```python
from build123d import *

# Parameters (mm, degrees)
BOSS_EXTRUDE5_DEPTH          = 2.760049195
CHAMFER1_SIZE                = 1.510362865
CHAMFER1_SIZE2               = 0.926037145
BOSS_EXTRUDE6_DEPTH          = 24
BOSS_EXTRUDE7_DEPTH          = 5
BOSS_EXTRUDE8_DEPTH          = 6
BOSS_EXTRUDE9_DEPTH          = 4
SKETCH28_W                   = 2.760049196
SKETCH28_H                   = 4
CUT_EXTRUDE3_DEPTH           = 8.878692186
BOSS_EXTRUDE10_DEPTH         = 4
SKETCH45_W                   = 2.760049196
SKETCH45_H                   = 4
CUT_EXTRUDE4_DEPTH           = 0.7448337
BOSS_EXTRUDE11_DEPTH         = 5
F_4_0_4_DIAMETER_HOLE2_D     = 4
F_4_0_4_DIAMETER_HOLE2_DEPTH = 2.760049195
SKETCH58_W                   = 2.6375
SKETCH58_H                   = 10
SKETCH60_W                   = 2.6375
SKETCH60_H                   = 38
HOLE6_D                      = 5.275
HOLE6_DEPTH                  = 46
F_3_0_3_DIAMETER_HOLE2_D     = 3
F_3_0_3_DIAMETER_HOLE2_DEPTH = 35
FILLET3_R                    = 2
FILLET4_R                    = 3


with BuildPart() as part:
    # Sketch17 → Boss-Extrude5 (new body)
    with BuildSketch(Plane(origin=(57.196631886, 0, 0), x_dir=(0, -1, 0), z_dir=(-1, 0, 0))):
        with BuildLine():
            Line((-38, -27.633835998), (-14, -27.633835998))
            ThreePointArc((-14, -27.633835998), (-12, -25.633835998), (-10, -27.633835998))
            Line((-10, -27.633835998), (-10, -9.028355512))
            Line((-10, -9.028355512), (-42, -9.028355512))
            Line((-42, -9.028355512), (-42, -27.633835998))
            ThreePointArc((-42, -27.633835998), (-40, -25.633835998), (-38, -27.633835998))
        make_face()
    extrude(amount=-BOSS_EXTRUDE5_DEPTH)

    # Chamfer1
    chamfer1_edges = [part.edges().sort_by_distance(p)[0] for p in [
        (59.956681082, 26, -9.028355512),
    ]]
    chamfer1_side = [part.faces().sort_by_distance(p)[0] for p in [
        (59.956681082, 26, -18.148814744),
    ]]
    chamfer(chamfer1_edges, length=CHAMFER1_SIZE, length2=CHAMFER1_SIZE2, reference=chamfer1_side[0])

    # Sketch18 → Boss-Extrude6 (add)
    with BuildSketch(Plane(origin=(0, 38, 0), x_dir=(1, 0, 0), z_dir=(0, 1, 0))):
        with BuildLine():
            Line((57.196631886, 27.633835998), (59.956681082, 27.633835998))
            Line((59.956681082, 27.633835998), (59.956681082, 37.518663649))
            ThreePointArc((59.956681082, 37.518663649), (52.044420209, 35.109942461), (57.196631886, 28.639971463))
            Line((57.196631886, 28.639971463), (57.196631886, 27.633835998))
        make_face()
    extrude(amount=-BOSS_EXTRUDE6_DEPTH)

    # Sketch19 → Boss-Extrude7 (add)
    with BuildSketch(Plane(origin=(0, 35, 0), x_dir=(1, 0, 0), z_dir=(0, 1, 0))):
        with BuildLine():
            Line((57.196631886, 15.88036097), (57.196631886, 23.207838196))
            add(Edge.make_bspline(
                [(55.511713205, 21.752088745), (56.732163203, 22.065636669), (57.196631886, 23.207838196)],
                knots=[0, 0, 0, 1, 1, 1], degree=2))
            ThreePointArc((55.511713205, 21.752088745), (53.511713205, 19.752088745), (55.511713205, 17.752088745))
            add(Edge.make_bspline(
                [(57.196631886, 15.88036097), (56.909946197, 17.31678815), (55.511713205, 17.752088745)],
                knots=[0, 0, 0, 1, 1, 1], degree=2))
        make_face()
    extrude(amount=-BOSS_EXTRUDE7_DEPTH)

    # Sketch20 → Boss-Extrude8 (add)
    with BuildSketch(Plane.XZ.offset(-10)):
        with BuildLine():
            Line((57.196631886, -28.639971463), (57.196631886, -9.028355512))
            Line((57.196631886, -9.028355512), (59.030643937, -9.028355512))
            Line((59.030643937, -9.028355512), (59.956681082, -10.538718377))
            Line((59.956681082, -10.538718377), (59.956681082, -37.518663649))
            ThreePointArc((59.956681082, -37.518663649), (52.044420209, -35.109942461), (57.196631886, -28.639971463))
        make_face()
    extrude(amount=BOSS_EXTRUDE8_DEPTH)

    # Sketch21 → Boss-Extrude9 (add)
    with BuildSketch(Plane.XZ.offset(-4)):
        Polygon((57.196631886, -27.895137764), (57.196631886, -9.028355512), (59.030643937, -9.028355512), (59.956681082, -10.538718377), (59.956681082, -27.895137764), (59.956681082, -28.639971463), (59.956681082, -37.518663649), (57.196631886, -37.518663649), (57.196631886, -28.639971463), align=None)
    extrude(amount=BOSS_EXTRUDE9_DEPTH)

    # Sketch28 → Cut-Extrude3 (cut)
    with BuildSketch(Plane(origin=(0, 0, -37.518663649), x_dir=(-1, 0, 0), z_dir=(0, 0, -1))):
        with Locations((-58.576656484, 2)):
            Rectangle(SKETCH28_W, SKETCH28_H)
    extrude(amount=-CUT_EXTRUDE3_DEPTH, mode=Mode.SUBTRACT)

    # Sketch36 → Boss-Extrude10 (add)
    with BuildSketch(Plane(origin=(0, 42, 0), x_dir=(1, 0, 0), z_dir=(0, 1, 0))):
        with BuildLine():
            Line((59.956681082, 37.518663649), (59.956681082, 10.538718377))
            Line((59.956681082, 10.538718377), (59.030643937, 9.028355512))
            Line((59.030643937, 9.028355512), (57.196631886, 9.028355512))
            Line((57.196631886, 9.028355512), (57.196631886, 28.639971463))
            ThreePointArc((57.196631886, 28.639971463), (52.044420209, 35.109942461), (59.956681082, 37.518663649))
        make_face()
    extrude(amount=BOSS_EXTRUDE10_DEPTH)

    # Sketch45 → Cut-Extrude4 (cut)
    with BuildSketch(Plane(origin=(0, 0, -28.639971463), x_dir=(-1, 0, 0), z_dir=(0, 0, -1))):
        with Locations((-58.576656484, 2)):
            Rectangle(SKETCH45_W, SKETCH45_H)
    extrude(amount=-CUT_EXTRUDE4_DEPTH, mode=Mode.SUBTRACT)

    # Sketch55 → Boss-Extrude11 (add)
    with BuildSketch(Plane(origin=(0, 46, 0), x_dir=(1, 0, 0), z_dir=(0, 1, 0))):
        Polygon((59.956681082, 10.538718377), (59.030643937, 9.028355512), (57.196631886, 9.028355512), (57.196631886, 27.895137764), (59.956681082, 27.895137764), align=None)
    extrude(amount=BOSS_EXTRUDE11_DEPTH)

    # Ø4.0 (4) Diameter Hole2
    with Locations(Plane.ZY.offset(-57.196631886)):
        with Locations((-22.895137764, 6), (-14.028355512, 6), (-14.028355512, 46), (-22.895137764, 46)):
            Hole(F_4_0_4_DIAMETER_HOLE2_D / 2, depth=F_4_0_4_DIAMETER_HOLE2_DEPTH)

    # Sketch58 → Hole4 (revolve, cut)
    with BuildSketch(Plane(origin=(56.81904117, 10, -33.625693603), x_dir=(0, 0, 1), z_dir=(1, 0, 0))):
        with Locations((1.31875, 5)):
            Rectangle(SKETCH58_W, SKETCH58_H)
    revolve(axis=Axis((56.81904117, -100, -33.625693603), (0, 1, 0)), mode=Mode.SUBTRACT)

    # Sketch60 → Hole5 (revolve, cut)
    with BuildSketch(Plane(origin=(56.81904117, 38, -33.625693603), x_dir=(0, 0, 1), z_dir=(1, 0, 0))):
        with Locations((1.31875, 19)):
            Rectangle(SKETCH60_W, SKETCH60_H)
    revolve(axis=Axis((56.81904117, -72, -33.625693603), (0, 1, 0)), mode=Mode.SUBTRACT)

    # Hole6
    with Locations(Plane(origin=(0, 46, 0), x_dir=(1, 0, 0), z_dir=(0, 1, 0))):
        with Locations((56.81904117, 33.625693603)):
            Hole(HOLE6_D / 2, depth=HOLE6_DEPTH)

    # Ø3.0 (3) Diameter Hole2
    with Locations(Plane(origin=(0, 35, 0), x_dir=(1, 0, 0), z_dir=(0, 1, 0))):
        with Locations((55.511713205, 19.752088745)):
            Hole(F_3_0_3_DIAMETER_HOLE2_D / 2, depth=F_3_0_3_DIAMETER_HOLE2_DEPTH)

    # Fillet3
    fillet3_edges = [part.edges().sort_by_distance(p)[0] for p in [
        (58.576656484, 46, -27.895137764),
        (58.576656484, 4, -27.895137764),
        (57.196631886, 26, -28.639971463),
    ]]
    fillet(fillet3_edges, radius=FILLET3_R)

    # Fillet4
    fillet4_edges = [part.edges().sort_by_distance(p)[0] for p in [
        (59.956681082, 26, -37.518663649),
        (59.956681082, 7, -37.518663649),
        (59.956681082, 44, -37.518663649),
    ]]
    fillet(fillet4_edges, radius=FILLET4_R)


solid = part.part
```
Work out the finished part from the listing and answer in its coordinate system (mm). A direction names the side the tool comes from. Round coordinates to 2 decimals unless told otherwise and drop trailing zeros. Write each loop counter-clockwise with the first axis right and the second up, starting at its lowest first coordinate (ties: lowest second). Pieces come first, ordered by that corner, then holes. Notation, with made-up numbers: (54, -10.5) -> (76, -10.5) arc R23 cw to (76, 1.5) -> close; hole circle Ø2 at (46.25, 30.25). An arc over 180 degrees is marked (long way). Write each question's results on one line, items separated by ' | '.
Q1. Straight lines are drawn through the part: line 1 along Y through (x, z) = (58.75, -31.5); line 2 along X through (y, z) = (20, -21.5); line 3 along Y through (x, z) = (59.25, -26). For each, find the intervals that lie inside material, in ascending order. Write a range as [from, to].
Data:
line 1: [4, 10], [14, 38], [42, 46] | line 2: [57.2, 59.96] | line 3: [0, 10.85], [13.15, 38.85], [41.15, 51]
Q2. Which of the six approach directions +Z, -Z, +X, -X, +Y, -Y give full straight-line access (tool end or side, diameter ignored) to faces 5 (the flat face through (59, 0, -18)), 6 (the flat face through (59, 1, -27.895)), 7 (the flat face through (54, 14, -33)), 8 (the flat face through (59, 49, -27.895))?
Data:
face 5: +Z, -Z, +X, -X, -Y | face 6: -Z, +X, -X, -Y | face 7: -Z, +X, -X | face 8: -Z, +X, -X, +Y
Q3. Section D-D, the plane x = 54.75 is taken. Give the number of separate pieces and of enclosed holes in the cut face, then the cut area to 3 significant figures.
Data:
separate pieces: 8 | enclosed holes: 0 | area: 204 mm^2
Q4. Flat-ended cylindrical pins translate along their axes: P1, Ø3, axis at x = 55, z = -20, coming from the +Y side; P2, Ø3.5, axis at y = 46, z = -22.9, coming from the +X side (1 decimal); P3, Ø6, axis at y = 34, z = -23.5, coming from the -X side; P4, Ø1.5, axis at y = 37.5, z = -15.5, coming from the -X side. Find the tip coordinate at first contact, or state that the pin passes through.
Data:
P1: y = 35 | P2: through | P3: x = 53.66 | P4: x = 57.2
Q5. Section A-A, the plane y = 6 is taken. Write down the section's boundary in (x, z) (1 decimal).
Data:
outline: (57.2, -38.6) arc R3 ccw to (60, -35.6) -> (60, -24.9) -> (57.2, -24.9) -> (57.2, -28.6) arc R5 ccw (long way) to start; (57.2, -20.9) -> (60, -20.9) -> (60, -16) -> (57.2, -16) -> close; (57.2, -12) -> (60, -12) -> (60, -10.5) -> (59, -9) -> (57.2, -9) -> close; hole circle Ø5.3 at (56.8, -33.6)
Q6. Determine the mould class of faces 1 (the cylindrical face through (55.214, 6.958, -35.719)), 2 (the flat face through (54, 42, -33)), 3 (the flat face through (57.197, 25, -19)), 4 (the cylindrical face through (55.214, 25.832, -35.719)) for opening direction X: released by +X, released by -X, zero draft, split by the parting line, or undercut.
Data:
face 1: undercut | face 2: zero draft | face 3: released by -X | face 4: undercut
Q7. Section B-B, the plane z = -31.75 is taken. Write down the section's boundary in (x, y), then the cut area to 3 significant figures.
Data:
outline: (52.18, 4) -> (54.96, 4) -> (54.96, 10) -> (52.18, 10) -> close; (52.18, 14) -> (54.96, 14) -> (54.96, 38) -> (52.18, 38) -> close; (52.18, 42) -> (54.96, 42) -> (54.96, 46) -> (52.18, 46) -> close; (58.67, 4) -> (59.96, 4) -> (59.96, 10) -> (58.67, 10) -> close; (58.67, 14) -> (59.96, 14) -> (59.96, 38) -> (58.67, 38) -> close; (58.67, 42) -> (59.96, 42) -> (59.96, 46) -> (58.67, 46) -> close | area: 138 mm^2
Q8. Section C-C, the plane z = -13.5 is taken. Write down the section's boundary in (x, y).
Data:
outline: (57.2, 0) -> (59.96, 0) -> (59.96, 4.07) -> (57.2, 4.07) -> close; (57.2, 7.93) -> (59.96, 7.93) -> (59.96, 44.07) -> (57.2, 44.07) -> close; (57.2, 47.93) -> (59.96, 47.93) -> (59.96, 51) -> (57.2, 51) -> close
